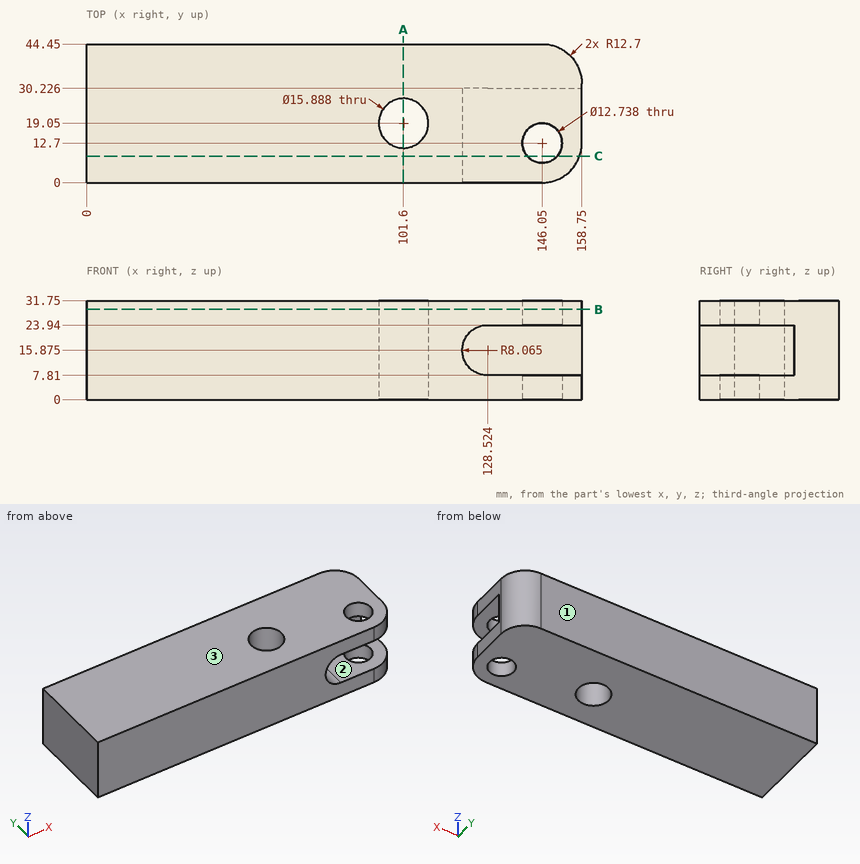
The drawing under review shows one solid part. Ordinate dimensions are in mm from its lowest x, y, z. Round coordinates to 2 decimals unless told otherwise and drop trailing zeros. Loops run counter-clockwise (first coordinate to the right, second up) from the corner with the lowest first, then second, coordinate; pieces in that order, holes last. Notation, with made-up numbers: M 65.5,15 L 77.5,15 A19 ccw 77.5,25 Z; hole C 72,47 d10. An arc over 180 degrees is marked long. Answer as CSV lines item,"result". Start each with the question number.
Item 1: Consider section A-A (x = 101.6). Write out the cut boundary in (y, z).
Item 2: Wall thickness on line 1 (Z direction, x = 150, y = 19); line 2 (Y direction, x = 101, z = 22); line 3 (Y direction, x = 146.05, z = 6): over which ranges is each line inside the solid? List them lowest first. Write a range as [from, to].
Item 3: Consider section B-B (z = 29). Write out the cut boundary in (x, y), then the cut area to 3 significant figures.
Item 4: Mouldability with a two-part tool opening along Z and no side actions: class the marked faces 1, 2 and 3 as released by +Z, released by -Z, zero draft, split by the parting line, or undercut.
Item 5: Consider section C-C (y = 8.5). State how many separate pieces and enclosed holes the cut face has, then the cut area to 3 significant figures.
Item 6: Insertion check: P1, Ø3, axis at y = 18, z = 13.5, coming from the +X side; P2, Ø13, axis at x = 132.5, z = 16, coming from the -Y side; P3, Ø3, axis at y = 37.5, z = 19.5, coming from the +X side. Each pin has a flat end and moves straight along its axis. Give the tip position at first contact, or say it passes through.
Answer:
1,outline,"M 0,0 L 11.11,0 L 11.11,31.75 L 0,31.75 Z; M 26.99,0 L 44.45,0 L 44.45,31.75 L 26.99,31.75 Z"
2,line 1,"z = [0, 7.81], [23.94, 31.75]"
2,line 2,"y = [0, 11.13], [26.97, 44.45]"
2,line 3,"y = [0, 6.33], [19.07, 44.45]"
3,outline,"M 0,0 L 146.05,0 A12.7 ccw 158.75,12.7 L 158.75,31.75 A12.7 ccw 146.05,44.45 L 0,44.45 Z; hole C 101.6,19.05 d15.89; hole C 146.05,12.7 d12.74"
3,area,"6,660 mm^2"
4,face 1,"zero draft"
4,face 2,"undercut"
4,face 3,"released by +Z"
5,separate pieces,"3"
5,enclosed holes,"0"
5,area,"4,290 mm^2"
6,P1,"stops at x = 121.45"
6,P2,"stops at y = 30.23"
6,P3,"stops at x = 158.02"
